Read the model definition and answer for the solid it produces. Units are mm, in the model's axes. Face numbers are marked on the shaded views. A direction names the side the tool comes from. Coordinates: 2 decimals unless noted, no trailing zeros. Order: outer loops, then holes, each group sorted by start corner. A loop starts at its lowest first (then second) coordinate and runs counter-clockwise, first axis right, second up. Notation, with made-up numbers: (43, 16) - (81, 16) arc R16 ccw to (81, 46) - close; hole circle Ø7 at (-26.5, -21.5). An arc over 180 degrees is marked (long way). Use one line per item in the form item = value. Start each with the question number.
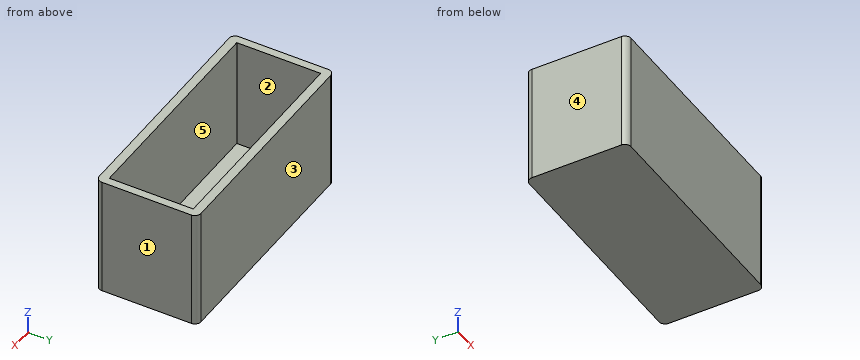
from build123d import *

# Parameters (mm, degrees)
F0_W     = 195
F0_H     = 85
F1_DEPTH = 100
F2_W     = 181.545526
F2_H     = 70.127204
F3_DEPTH = 93
F4_R     = 5.08


with BuildPart() as f1:
    # F0 (on Top) → F1 (new body)
    with BuildSketch(Plane.XY):
        Rectangle(F0_W, F0_H)
    extrude(amount=F1_DEPTH)

    # F2 (on face) → F3 (cut)
    with BuildSketch(Plane.XY.offset(100)):
        Rectangle(F2_W, F2_H)
    extrude(amount=-F3_DEPTH, mode=Mode.SUBTRACT)

    # F4
    f4_edges = [f1.edges().sort_by_distance(p)[0] for p in [
        (97.5, -42.5, 50),
        (97.5, 42.5, 50),
        (-97.5, -42.5, 50),
        (-97.5, 42.5, 50),
    ]]
    fillet(f4_edges, radius=F4_R)


solid = f1.part
Q1. Given P1, Ø2, axis at x = -7.5, y = 11.5, coming from the +Z side, flat-ended and moving along its own axis, determine where the tip first touches the part or whether it passes through.
Q2. A cutting plane is placed at A-A (z = 59). Give the vertices of the cut face in (x, y).
Q3. A cutting plane is placed at C-C (y = -6). Give the vertices of the cut face in (x, z).
Q4. Consider probe 1 along Y at (x, z) = (-89, 14); probe 2 along X at (y, z) = (-33, 29); probe 3 along Z at (x, y) = (80, -25.5). Determine where each line is inside the solid, lowest interval first.
Q5. Which of the six approach directions +Z, -Z, +X, -X, +Y, -Y give full straight-line access (tool end or side, diameter ignored) to the marked faces 4 and 5?
Q6. For a pull along Y with two mould halves and no side action, classify the marked faces 1, 2 and 3 as +Y half, -Y half, draft (parallel to the pull), parting line (faces both ways), or undercut.
Q7. A cutting plane is placed at B-B (x = 1.5). Give the vertices of the cut face in (y, z), then the cut area to 3 significant figures.
Result sheet:
q1.P1 = 7
q2.outline = (-97.5, -37.42) arc R5.08 ccw to (-92.42, -42.5) - (92.42, -42.5) arc R5.08 ccw to (97.5, -37.42) - (97.5, 37.42) arc R5.08 ccw to (92.42, 42.5) - (-92.42, 42.5) arc R5.08 ccw to (-97.5, 37.42) - close; hole (-90.77, -35.06) - (90.77, -35.06) - (90.77, 35.06) - (-90.77, 35.06) - close
q3.outline = (-97.5, 0) - (97.5, 0) - (97.5, 100) - (90.77, 100) - (90.77, 7) - (-90.77, 7) - (-90.77, 100) - (-97.5, 100) - close
q4.probe_1 = -42.5 to -35.06, 35.06 to 42.5
q4.probe_2 = -97.5 to -90.77, 90.77 to 97.5
q4.probe_3 = 0 to 7
q5.face_4 = +Z, -Z, -X, +Y, -Y
q5.face_5 = +Z
q6.face_1 = draft
q6.face_2 = undercut
q6.face_3 = +Y half
q7.outline = (-42.5, 0) - (42.5, 0) - (42.5, 100) - (35.06, 100) - (35.06, 7) - (-35.06, 7) - (-35.06, 100) - (-42.5, 100) - close
q7.area = 1,980 mm^2
